Geometry: final body of the model. Coordinates: model frame, mm. Give positions to 0.01 mm unless a question says otherwise; leave off trailing zeros. Write each loop counter-clockwise with the first axis right and the second up, starting at its lowest first coordinate (ties: lowest second). Pieces come first, ordered by that corner, then holes.
Q1. Section B-B (z = 5.25). Return the cut outline in (x, y), plus the area to 3 significant figures.
Q2. Section A-A (x = -100). Return the cut outline in (y, z).
Q3. Line query: line 1 (X direction, y = 15.25, z = 10.75); line 2 (Y direction, x = -100, z = 12); line 3 (Y direction, x = 3, z = 12.5). Output: solid intervals per line, ascending.
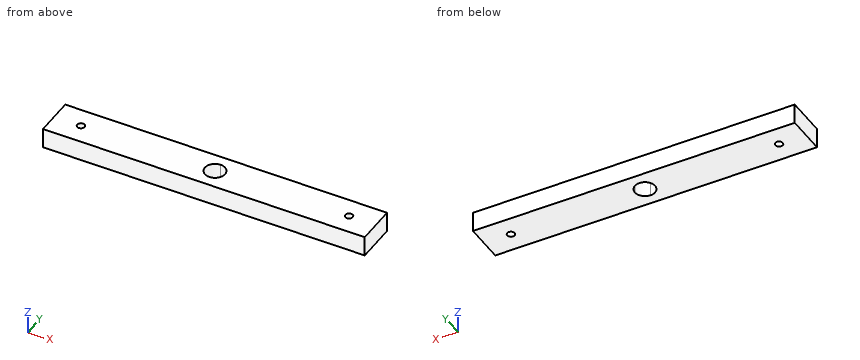
from build123d import *

# Parameters (mm, degrees)
RESSALTO_EXTRUS_O1_DEPTH = 15
CORTE_EXTRUS_O1_DEPTH    = 15
ESBO_O3_R                = 2.75
CORTE_EXTRUS_O2_DEPTH    = 50


with BuildPart() as part:
    # Esboço1 → Ressalto-extrusão1 (new body)
    with BuildSketch(Plane.XY):
        Polygon((100, 0), (-100, 0), (-120, 0), (-120, 30), (-100, 30), (100, 30), (120, 30), (120, 0), align=None)
    extrude(amount=RESSALTO_EXTRUS_O1_DEPTH)

    # Esboço2 → Corte-extrusão1 (cut)
    with BuildSketch(Plane.XY.offset(15)):
        with BuildLine():
            ThreePointArc((7.5, 15), (5.303300859, 20.303300859), (0, 22.5))
            Line((0, 22.5), (0, 7.5))
            ThreePointArc((0, 7.5), (5.303300859, 9.696699141), (7.5, 15))
        make_face()
        with BuildLine():
            Line((0, 7.5), (0, 22.5))
            ThreePointArc((0, 22.5), (-7.5, 15), (0, 7.5))
        make_face()
    extrude(amount=-CORTE_EXTRUS_O1_DEPTH, mode=Mode.SUBTRACT)

    # Esboço3 → Corte-extrusão2 (cut)
    with BuildSketch(Plane.XY.offset(15)):
        with Locations((-100, 15)):
            Circle(ESBO_O3_R)
        with Locations((100, 15)):
            Circle(ESBO_O3_R)
    extrude(amount=-CORTE_EXTRUS_O2_DEPTH, mode=Mode.SUBTRACT)


solid = part.part
Computed:
1. outline: (-120, 0) - (120, 0) - (120, 30) - (-120, 30) - close; hole circle Ø5.5 at (-100, 15); hole circle Ø15 at (0, 15); hole circle Ø5.5 at (100, 15)
1. area: 6,980 mm2
2. outline: (0, 0) - (12.25, 0) - (12.25, 15) - (0, 15) - close; (17.75, 0) - (30, 0) - (30, 15) - (17.75, 15) - close
3. line 1: x = -120 to -102.74, -97.26 to -7.5, 7.5 to 97.26, 102.74 to 120
3. line 2: y = 0 to 12.25, 17.75 to 30
3. line 3: y = 0 to 8.13, 21.87 to 30
